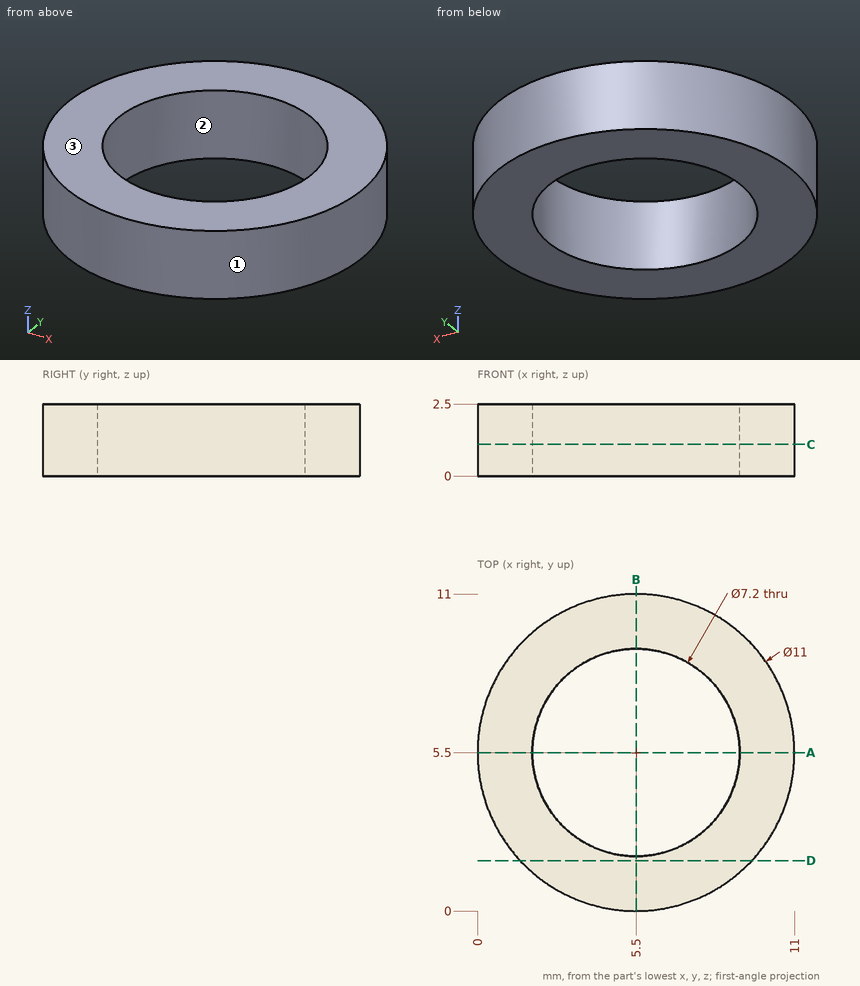
Design review of the part shown in the three views and the two pictorial views. Dimensions are in mm from the part's minimum x, y and z. Round coordinates to 2 decimals unless told otherwise and drop trailing zeros. Write each loop counter-clockwise with the first axis right and the second up, starting at its lowest first coordinate (ties: lowest second). Pieces come first, ordered by that corner, then holes. Notation, with made-up numbers: M -36.5,49 L -5.5,49 A18 cw -5.5,61 Z; hole C -18,-35 d2. An arc over 180 degrees is marked long. Use a Markdown table: item, result. Add a question column.
Q1. We need section A-A, the plane y = 5.5. State the section outline as (x, z) points, plus the area to 3 significant figures.
Q2. We need section D-D, the plane y = 1.75. State the section outline as (x, z) points.
Q3. We need section C-C, the plane z = 1.1. State the section outline as (x, y) points.
Q4. To check wall thickness, follow line 1 (Y direction, x = 5.5, z = 2); line 2 (Y direction, x = 2.75, z = 0.65); line 3 (X direction, y = 8, z = 0.45). State the ranges of each line that lie inside material, in increasing order.
Q5. The part is to be moulded in two halves that separate along X. For the marked faces 1, 2 and 3, say which applies: pulls with the +X half, pulls with the -X half, needs draft (parallel to the pull), parting line crosses it, or undercut.
Q6. Insertion check: pin 1 (1.5 mm diameter, centred on x = 3.5, z = 0.5, fed in from +Y). The pin has a flat end and moves straight along its axis. Give the tip position at first contact, or say it passes through.
Findings below:
| question | item | result |
|---|---|---|
| 1 | outline | M 0,0 L 1.9,0 L 1.9,2.5 L 0,2.5 Z; M 9.1,0 L 11,0 L 11,2.5 L 9.1,2.5 Z |
| 1 | area | 9.50 mm² |
| 2 | outline | M 1.48,0 L 9.52,0 L 9.52,2.5 L 1.48,2.5 Z |
| 3 | outline | C 5.5,5.5 d11; hole C 5.5,5.5 d7.2 |
| 4 | line 1 | y = 0 to 1.9, 9.1 to 11 |
| 4 | line 2 | y = 0.74 to 3.18, 7.82 to 10.26 |
| 4 | line 3 | x = 0.6 to 2.91, 8.09 to 10.4 |
| 5 | face 1 | parting line crosses it |
| 5 | face 2 | undercut |
| 5 | face 3 | needs draft |
| 6 | pin 1 | stops at y = 10.86 |
